Verification items for the finished model (mm, model axes). Face numbers are marked on the shaded views. Coordinates: 2 decimals unless noted, no trailing zeros. Order: outer loops, then holes, each group sorted by start corner. A loop starts at its lowest first (then second) coordinate and runs counter-clockwise, first axis right, second up. Notation, with made-up numbers: (-8, -12) -> (20, -12) arc R28 cw to (20, 7) -> close; hole circle Ø6 at (23.5, -16.75). An arc over 180 degrees is marked (long way). Write item = value, one per line. Start each with the question number.
1. Cross-section at C-C on x = 0. Record the cut outline in (y, z).
2. Thickness scan on line 1 along Y through (x, z) = (0, 8.35); line 2 along X through (y, z) = (-8, 9.25); line 3 along X through (y, z) = (-15, 9). Record the ranges inside material, lowest first. Write a range as from..to.
3. Cross-section at A-A on z = 8.5. Record the cut outline in (x, y).
4. Cross-section at B-B on y = 0. Record the cut outline in (x, z), plus the area to 3 significant figures.
5. Cross-section at D-D on y = 22. Record the cut outline in (x, z).
6. Release check for a two-part mould opening along Y. For the marked faces 1, 2, 3 and 4 record: +Y half, -Y half, draft (parallel to the pull), parting line (faces both ways), or undercut.
7. Go/stop test with flat-tipped pins: P1, Ø5, axis at y = 33.5, z = 1.5, coming from the +X side; P2, Ø5.5, axis at x = 1.5, y = 0, coming from the +Z side; P3, Ø5, axis at y = -10.5, z = 4.5, coming from the +X side. Record where each tip stops, or that it passes through.
from build123d import *

# Parameters (mm, degrees)
EXTRUDE_1_DEPTH     = 10
SKETCH_2_R          = 4.468909074
SKETCH_2_R_2        = 4.108968286
CUT_EXTRUDE_1_DEPTH = 111.460779809
SKETCH_3_R          = 50.74720983
SKETCH_3_R_2        = 43.56554387
CUT_EXTRUDE_3_DEPTH = 4
SKETCH_4_R          = 9.24493497
CUT_EXTRUDE_4_DEPTH = 4
SKETCH_5_R          = 18.201318997
CUT_EXTRUDE_5_DEPTH = 5


with BuildPart() as part:
    # 草图1 → 凸台-拉伸1 (new body)
    with BuildSketch(Plane.XY):
        with BuildLine():
            Line((-89.657800503, -43.044325296), (-15.652055073, -61.790580648))
            ThreePointArc((-15.652055073, -61.790580648), (63.74215783, 0), (-15.652055073, 61.790580648))
            Line((-15.652055073, 61.790580648), (-89.657800503, 43.044325296))
            Line((-89.657800503, 43.044325296), (-89.657800503, 32.044242854))
            ThreePointArc((-89.657800503, 32.044242854), (-89.034636537, 28.569340555), (-87.242811306, 25.527525035))
            ThreePointArc((-87.242811306, 25.527525035), (-77.782727423, 0), (-87.242811306, -25.527525035))
            ThreePointArc((-87.242811306, -25.527525035), (-89.034636537, -28.569340555), (-89.657800503, -32.044242854))
            Line((-89.657800503, -32.044242854), (-89.657800503, -43.044325296))
        make_face()
    extrude(amount=EXTRUDE_1_DEPTH)

    # 草图2 → 切除-拉伸1 (cut, through all)
    with BuildSketch(Plane.XY.offset(10)):
        with Locations((-80.107707578, 35.677130973)):
            Circle(SKETCH_2_R)
        with Locations(Location((-80.107707578, -35.677130973, 0), (0, 0, 180))):
            Circle(SKETCH_2_R)
        with Locations((56.919679182, 0)):
            Circle(SKETCH_2_R_2)
    extrude(amount=-CUT_EXTRUDE_1_DEPTH, mode=Mode.SUBTRACT)

    # 草图3 → 切除-拉伸3 (cut)
    with BuildSketch(Plane.XY.offset(10)):
        Circle(SKETCH_3_R)
        Circle(SKETCH_3_R_2, mode=Mode.SUBTRACT)
    extrude(amount=-CUT_EXTRUDE_3_DEPTH, mode=Mode.SUBTRACT)

    # 草图4 → 切除-拉伸4 (cut)
    with BuildSketch(Plane.XY.offset(10)):
        Circle(SKETCH_4_R)
    extrude(amount=-CUT_EXTRUDE_4_DEPTH, mode=Mode.SUBTRACT)

    # 草图5 → 切除-拉伸5 (cut)
    with BuildSketch(Plane(origin=(0, 0, 0), x_dir=(-1, 0, 0), z_dir=(0, 0, -1))):
        Circle(SKETCH_5_R)
    extrude(amount=-CUT_EXTRUDE_5_DEPTH, mode=Mode.SUBTRACT)


solid = part.part
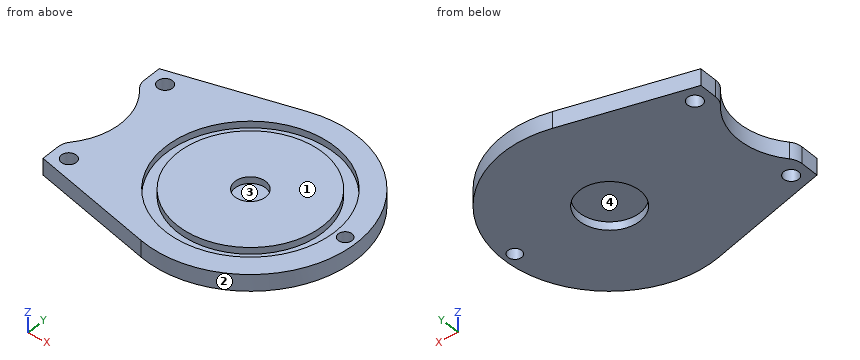
Worked out:
q1.outline = (-63.74, 0) -> (-18.2, 0) -> (-18.2, 5) -> (18.2, 5) -> (18.2, 0) -> (63.74, 0) -> (63.74, 10) -> (50.75, 10) -> (50.75, 6) -> (43.57, 6) -> (43.57, 10) -> (9.24, 10) -> (9.24, 6) -> (-9.24, 6) -> (-9.24, 10) -> (-43.57, 10) -> (-43.57, 6) -> (-50.75, 6) -> (-50.75, 10) -> (-63.74, 10) -> close
q2.line_1 = -63.74..-50.75, -43.57..-9.24, 9.24..43.57, 50.75..63.74
q2.line_2 = -78.61..-50.11, -42.82..-4.63, 4.63..42.82, 50.11..63.24
q2.line_3 = -80.77..-48.48, -40.9..40.9, 48.48..61.95
q3.outline = (-89.66, -43.04) -> (-15.65, -61.79) arc R63.74 ccw (long way) to (-15.65, 61.79) -> (-89.66, 43.04) -> (-89.66, 32.04) arc R10 ccw to (-87.24, 25.53) arc R39.17 cw to (-87.24, -25.53) arc R10 ccw to (-89.66, -32.04) -> close; circle Ø87.13 at (0, 0); hole circle Ø8.94 at (-80.11, -35.68); hole circle Ø8.94 at (-80.11, 35.68); hole circle Ø101.49 at (0, 0); hole circle Ø18.49 at (0, 0); hole circle Ø8.22 at (56.92, 0)
q4.outline = (-77.78, 0) -> (-18.2, 0) -> (-18.2, 5) -> (18.2, 5) -> (18.2, 0) -> (52.81, 0) -> (52.81, 10) -> (50.75, 10) -> (50.75, 6) -> (43.57, 6) -> (43.57, 10) -> (9.24, 10) -> (9.24, 6) -> (-9.24, 6) -> (-9.24, 10) -> (-43.57, 10) -> (-43.57, 6) -> (-50.75, 6) -> (-50.75, 10) -> (-77.78, 10) -> close; (61.03, 0) -> (63.74, 0) -> (63.74, 10) -> (61.03, 10) -> close
q4.area = 1,020 mm²
q5.outline = (-84.54, 0) -> (59.83, 0) -> (59.83, 10) -> (45.73, 10) -> (45.73, 6) -> (37.6, 6) -> (37.6, 10) -> (-37.6, 10) -> (-37.6, 6) -> (-45.73, 6) -> (-45.73, 10) -> (-84.54, 10) -> close
q6.face_1 = draft
q6.face_2 = parting line
q6.face_3 = undercut
q6.face_4 = undercut
q7.P1 = 55.7
q7.P2 = 6
q7.P3 = 63.24
